```python
from build123d import *

# Parameters (mm, degrees)
SKETCH_1_R      = 1
EXTRUDE_1_DEPTH = 0.5
CHAMFER_1_SIZE  = 0.85
SCALE_1_SCALE   = 1.08


with BuildPart() as part:
    # Эскиз1 → Бобышка-Вытянуть1 (new body)
    with BuildSketch(Plane.XY):
        with BuildLine():
            Line((-15.6, 13), (-15.6, -13))
            ThreePointArc((-15.6, -13), (-14.838477631, -14.838477631), (-13, -15.6))
            Line((-13, -15.6), (-12.5, -15.6))
            Line((-12.5, -15.6), (-4.5, -15.6))
            ThreePointArc((-4.5, -15.6), (-3.01507576, -16.21507576), (-2.4, -17.7))
            Line((-2.4, -17.7), (-2.4, -18.2))
            ThreePointArc((-2.4, -18.2), (0, -20.6), (2.4, -18.2))
            Line((2.4, -18.2), (2.4, -17.7))
            ThreePointArc((2.4, -17.7), (3.01507576, -16.21507576), (4.5, -15.6))
            Line((4.5, -15.6), (12.5, -15.6))
            Line((12.5, -15.6), (13, -15.6))
            ThreePointArc((13, -15.6), (14.838477631, -14.838477631), (15.6, -13))
            Line((15.6, -13), (15.6, 13))
            ThreePointArc((15.6, 13), (14.838477631, 14.838477631), (13, 15.6))
            Line((13, 15.6), (12.5, 15.6))
            Line((12.5, 15.6), (4.5, 15.6))
            ThreePointArc((4.5, 15.6), (3.01507576, 16.21507576), (2.4, 17.7))
            Line((2.4, 17.7), (2.4, 18.2))
            ThreePointArc((2.4, 18.2), (0, 20.6), (-2.4, 18.2))
            Line((-2.4, 18.2), (-2.4, 17.7))
            ThreePointArc((-2.4, 17.7), (-3.01507576, 16.21507576), (-4.5, 15.6))
            Line((-4.5, 15.6), (-12.5, 15.6))
            Line((-12.5, 15.6), (-13, 15.6))
            ThreePointArc((-13, 15.6), (-14.838477631, 14.838477631), (-15.6, 13))
        make_face()
        with Locations((0, 18.2)):
            Circle(SKETCH_1_R, mode=Mode.SUBTRACT)
        with Locations(Location((0, -18.2, 0), (0, 0, 180))):
            Circle(SKETCH_1_R, mode=Mode.SUBTRACT)
    extrude(amount=EXTRUDE_1_DEPTH)

    # Фаска1
    # the kernel refuses this chamfer: 0.85 mm, written as the material it takes off along each edge
    with BuildSketch(Plane(origin=(0, -18.2, 0.5), x_dir=(-1, 0, 0), z_dir=(0, 1, 0))) as chamfer_1_piece_1:
        Polygon((1 + CHAMFER_1_SIZE, 0), (1, -CHAMFER_1_SIZE), (1, 0), align=None)
    revolve(axis=Axis((0, -18.2, 0.5), (0, 0, 1)), mode=Mode.SUBTRACT)
    with BuildSketch(Plane(origin=(0, 18.2, 0.5), x_dir=(1, 0, 0), z_dir=(0, -1, 0))) as chamfer_1_piece_2:
        Polygon((1 + CHAMFER_1_SIZE, 0), (1, -CHAMFER_1_SIZE), (1, 0), align=None)
    revolve(axis=Axis((0, 18.2, 0.5), (0, 0, 1)), mode=Mode.SUBTRACT)


with BuildPart() as part_1:
    # Масштаб1: scaled about (0, 0, 0.249580392)
    add(part.part.scale(SCALE_1_SCALE).moved(Location((0, 0, -0.019966431))))


solid = part_1.part
```
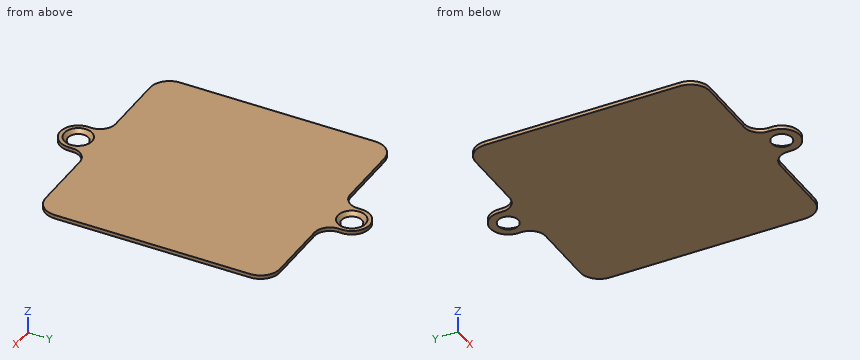
Source: CAD feature listing. Evaluate the final solid. Frame: model axes, mm. Give positions to 0.01 mm unless a question says otherwise; leave off trailing zeros. Loops run counter-clockwise (first coordinate to the right, second up) from the corner with the lowest first, then second, coordinate; pieces in that order, holes last. Notation, with made-up numbers: (9, 70.25) -> (56, 70.25) arc R34 ccw to (56, 104.25) -> close; hole circle Ø5 at (-18, 40.5). An arc over 180 degrees is marked (long way). Put each result on its own line as item: value. Start each with the question number.
1) Cut plane B-B (x = 0). Return loops of the section in (y, z).
2) Cut plane C-C (x = 13.5). Return loops of the section in (y, z), then the cut area to 3 significant figures.
3) Material intervals for probe 1 along Y at (x, z) = (-1, 0.45); probe 2 along Y at (x, z) = (-13.5, 0.4); probe 3 along X at (y, z) = (-19, 0.4), sorted ascending.
4) Cut plane A-A (z = 0.1). Return loops of the section in (x, y).
Results are:
1. outline: (-22.25, -0.02) -> (-21.11, -0.02) -> (-21.65, 0.52) -> (-22.25, 0.52) -> close; (-18.2, -0.02) -> (18.2, -0.02) -> (17.66, 0.52) -> (-17.66, 0.52) -> close; (21.11, -0.02) -> (22.25, -0.02) -> (22.25, 0.52) -> (21.65, 0.52) -> close
2. outline: (-16.85, -0.02) -> (16.85, -0.02) -> (16.85, 0.52) -> (-16.85, 0.52) -> close
2. area: 18.2 mm2
3. probe 1: y = -22.05 to -21.3, -18.01 to 18.01, 21.3 to 22.05
3. probe 2: y = -16.85 to 16.85
3. probe 3: x = -2.59 to -1.76, 1.76 to 2.59
4. outline: (-16.85, -14.04) arc R2.81 ccw to (-14.04, -16.85) -> (-4.86, -16.85) arc R2.27 cw to (-2.59, -19.12) -> (-2.59, -19.66) arc R2.59 ccw to (2.59, -19.66) -> (2.59, -19.12) arc R2.27 cw to (4.86, -16.85) -> (14.04, -16.85) arc R2.81 ccw to (16.85, -14.04) -> (16.85, 14.04) arc R2.81 ccw to (14.04, 16.85) -> (4.86, 16.85) arc R2.27 cw to (2.59, 19.12) -> (2.59, 19.66) arc R2.59 ccw to (-2.59, 19.66) -> (-2.59, 19.12) arc R2.27 cw to (-4.86, 16.85) -> (-14.04, 16.85) arc R2.81 ccw to (-16.85, 14.04) -> close; hole circle Ø3.16 at (0, -19.66); hole circle Ø3.16 at (0, 19.66)
